from build123d import *

# Parameters (mm, degrees)
F0_W      = 101.6
F0_H      = 12.7
F1_DEPTH  = 19.05
F2_W      = 6.35
F2_H      = 9.525
F3_DEPTH  = 25.4
F4_R      = 3.175
F6_DEPTH  = 12.7
F7_W      = 20.32
F7_H      = 12.7
F8_DEPTH  = 6.35
F9_R      = 4.7625
F9_R_2    = 3.175
F10_DEPTH = 3.175
F11_DEPTH = 6.35


with BuildPart() as f1:
    # F0 (on Front) → F1 (new body)
    with BuildSketch(Plane.XZ):
        with Locations((50.8, 6.35)):
            Rectangle(F0_W, F0_H)
    extrude(amount=F1_DEPTH)

    # F2 (on face) → F3 (cut)
    with BuildSketch(Plane.XY.offset(12.7)):
        with Locations((3.175, -4.7625)):
            Rectangle(F2_W, F2_H)
    extrude(amount=-F3_DEPTH, mode=Mode.SUBTRACT)

    # F4 (on face) → F6 (cut)
    with BuildSketch(Plane(origin=(0, 0, 0), x_dir=(-1, 0, 0), z_dir=(0, 1, 0))):
        with Locations((-12.7, 6.35)):
            Circle(F4_R)
    extrude(amount=-F6_DEPTH, mode=Mode.SUBTRACT)

    # F7 (on face) → F8 (join)
    with BuildSketch(Plane(origin=(0, 0, 0), x_dir=(-1, 0, 0), z_dir=(0, 1, 0))):
        with Locations((-8.89, 6.35)):
            Rectangle(F7_W, F7_H)
    extrude(amount=F8_DEPTH)

    # F9 (on face) → F10 (cut)
    with BuildSketch(Plane(origin=(0, 6.35, 0), x_dir=(-1, 0, 0), z_dir=(0, 1, 0))):
        with Locations((-12.7, 6.35)):
            Circle(F9_R)
        with Locations((-12.7, 6.35)):
            Circle(F9_R_2, mode=Mode.SUBTRACT)
    extrude(amount=-F10_DEPTH, mode=Mode.SUBTRACT)

    # F11 (cut): a face of the model
    f11_faces = [f1.faces().sort_by_distance(p)[0] for p in [
        (12.7, 6.35, 6.35),
    ]]
    extrude(f11_faces, amount=-F11_DEPTH, mode=Mode.SUBTRACT)


solid = f1.part
CAD build for the part. Positions are in the model's coordinates, mm. A direction names the side the tool comes from. Round coordinates to 2 decimals unless told otherwise and drop trailing zeros. Loops run counter-clockwise (first coordinate to the right, second up) from the corner with the lowest first, then second, coordinate; pieces in that order, holes last.
(1) Wall check: line 1 along Z through (x, y) = (12.7, -4.75) (3 decimals); line 2 along Z through (x, y) = (12.7, 5.05); line 3 along Y through (x, z) = (23, 12.25). Give the ranges that are in metal, low to high.
(2) Drop flat-ended pins along their axis: pin 1 (5 mm diameter, centred on y = -12, z = 4, fed in from -X); pin 2 (5 mm diameter, centred on x = 65, z = 9, fed in from +Y); pin 3 (1.9 mm diameter, centred on y = 3, z = 5.5, fed in from +X). Give the stop position or say it passes through.
(3) Cut at D-D (y = -6). Give the cut face in (x, z) (3 decimals).
(4) Two-plate mould, pull along Z, no slides. Class faces 4 (the flat face through (51, -9, 12.7)), 5 (the flat face through (12, 3.175, 3)), 6 (the cylindrical face through (10.993, -4.651, 9.027)), 7 (the flat face through (7, 6.35, 6)): +Z half, -Z half, draft (parallel to the pull), parting line (faces both ways), or undercut.
(5) Cut at C-C (y = -11.5). Give the cut face in (x, z) (3 decimals), plus the area to 3 significant figures.
(6) Which spindle directions (+Z, -Z, +X, -X, +Y, -Y) get a long thin tool onto all of the face, cutting with end or side? Do faces 1 (the flat face through (13, -12.7, 6)), 2 (the flat face through (6.35, -5, 6)), 3 (the flat face through (60, 0, 6)). Say none if no direction does.
Findings below:
1. line 1: z = 0 to 3.175, 9.525 to 12.7
1. line 2: z = 0 to 1.59, 11.11 to 12.7
1. line 3: y = -19.05 to 0
2. pin 1: stops at x = 0
2. pin 2: stops at y = 0
2. pin 3: stops at x = 19.05
3. outline: (6.35, 0) - (101.6, 0) - (101.6, 12.7) - (6.35, 12.7) - close; hole circle Ø6.35 at (12.7, 6.35)
4. face 4: +Z half
4. face 5: undercut
4. face 6: undercut
4. face 7: draft
5. outline: (0, 0) - (101.6, 0) - (101.6, 12.7) - (0, 12.7) - close; hole circle Ø6.35 at (12.7, 6.35)
5. area: 1,260 mm2
6. face 1: +Y
6. face 2: +Z, -Z, -X
6. face 3: +Z, -Z, +X, +Y
